Here's how the part is built. I have some questions about the finished solid (model axes, mm). A direction names the side the tool comes from. Give positions to 0.01 mm unless a question says otherwise; leave off trailing zeros. Return JSON: item names as keys, results as strings. Group by question number.
(1) On a 3-axis mill with a long thin cutter (end or side, diameter ignored), from which of +Z, -Z, +X, -X, +Y, -Y can I reach the whole of each face in a straight line? I mean faces 1 (the cylindrical face through (35.41, -1.73, -7.81)), 2 (the conical face through (2.54, 8.13, 2.56)). Say none if no direction works.
(2) For P1, Ø8, axis at x = 32.5, y = 3.5, coming from the -Z side; P2, Ø8, axis at x = 23.5, z = -5, coming from the +Y side; P3, Ø8, axis at x = 34, z = -6.5, coming from the -Y side, each with a flat end and sliding along its axis, tell me the tip position at first contact or that it passes through.
(3) I need wall thicknesses on probe 1 along X at (y, z) = (3.5, 7.5); probe 2 along Y at (x, z) = (34.5, -4); probe 3 along Z at (x, y) = (18, -1.5). Which ranges of each line are inside material? Lowest first, please. Write a range as [from, to].
```python
from build123d import *

# Parameters (mm, degrees)
THDSCHPAT_COUNT = 19
THDSCHPAT_PITCH = 1.952710494


with BuildPart() as part:
    # BodySke → Body (revolve)
    with BuildSketch(Plane.XY):
        with BuildLine():
            Line((0, 0), (0, 8.5))
            Line((0, 8.5), (5, 8.55))
            Line((5, 8.55), (5, 8))
            Line((5, 8), (47, 8))
            Line((47, 8), (49, 6))
            Line((49, 6), (48.905973721, 6))
            ThreePointArc((48.905973721, 6), (49.724257132, 3.049462801), (50, 0))
            Line((50, 0), (0, 0))
        make_face()
    revolve(axis=Axis((-8.740321592, 0, 0), (1, 0, 0)))

    # ThdSchSke → ThreadSchematic (revolve, cut)
    with BuildSketch(Plane.XY):
        Polygon((11, 6.8985), (10.19371102, 8.05), (11.80628898, 8.05), align=None)
    threadschematic = revolve(axis=Axis((112.074944318, 0, 0), (1, 0, 0)), mode=Mode.SUBTRACT)

    # ThdSchPat: ThreadSchematic ×19
    with Locations(*[(i * THDSCHPAT_PITCH, 0, 0) for i in range(1, THDSCHPAT_COUNT)]):
        add(threadschematic, mode=Mode.SUBTRACT)


solid = part.part
```
Values:
{
 "1": {"face 1": "+X", "face 2": "-X"},
 "2": {"P1": "z = -8", "P2": "y = 7.94", "P3": "y = -7.59"},
 "3": {"probe 1": "[0, 5]", "probe 2": "[-5.74, 5.74]", "probe 3": "[-7.86, 7.86]"}
}
